Autodesk Inventor part; units mm, degrees
ref_plane "Work Plane1" through (0, 0, 10) normal (0, 0, 1) x (1, 0, 0)
ref_plane "YZ Plane" through (0, 0, 0) normal (1, 0, 0) x (0, 1, 0)
ref_plane "XZ Plane" through (0, 0, 0) normal (0, 1, 0) x (-1, 0, 0)
ref_plane "Work Plane1" through (0, 0, 10) normal (0, 0, 1) x (1, 0, 0)
sketch "Sketch1" plane through (0, 0, 10) normal (0, 0, 1) x (1, 0, 0)
  line L0 (-4.0299, -0.3538) -> (-2.2322, 1.4439) construction
  arc A0 (-1.4439, 2.2322) -> (-2.2322, 1.4439) centre (-0.9299, 0.9299) ccw construction
  line L1 (-1.4439, 2.2322) -> (0.3538, 4.0299) construction
  line L2 (-37.8299, 42.8299) -> (-37.8299, 37.8299) construction
  line L3 (-37.8299, 37.8299) -> (-42.9208, 37.8299) construction
  line L4 (-37.8299, 42.2137) -> (-37.8299, 45.8299) construction
  line L5 (-37.8299, 45.8299) -> (-4.0299, 45.8299) construction
  line L6 (-4.0299, 45.8299) -> (-4.0299, 42.2137) construction
  line L7 (-4.0299, 4.0299) -> (0.3538, 4.0299)
  circle A1 centre (-20.9299, 20.9299) radius 17.5
  line L8 (-20.9299, 58.9723) -> (17.1124, 20.9299) construction
  line L9 (17.1124, 20.9299) -> (-20.9299, -17.1124) construction
  line L10 (-20.9299, -17.1124) -> (-58.9723, 20.9299) construction
  line L11 (-58.9723, 20.9299) -> (-20.9299, 58.9723) construction
  line L12 (-20.9299, 58.9723) -> (-20.9299, -17.1124) construction
  line L13 (17.1124, 20.9299) -> (-58.9723, 20.9299) construction
  line L14 (-20.9299, 58.9723) -> (32.8701, 58.9723) construction
  line L15 (-43.4299, 43.4299) -> (1.5701, 43.4299) construction
  line L16 (1.5701, 43.4299) -> (1.5701, -1.5701) construction
  line L17 (1.5701, -1.5701) -> (-43.4299, -1.5701) construction
  line L18 (-43.4299, -1.5701) -> (-43.4299, 43.4299) construction
  line L19 (-43.4299, 43.4299) -> (1.5701, -1.5701) construction
  line L20 (1.5701, 43.4299) -> (-43.4299, -1.5701) construction
  line L21 (-43.4299, 5.3876) -> (-43.4299, 36.4723)
  line L22 (-43.4299, 36.4723) -> (-36.4723, 43.4299)
  line L23 (-36.4723, 43.4299) -> (-5.3876, 43.4299)
  line L24 (-5.3876, 43.4299) -> (1.5701, 36.4723)
  line L25 (1.5701, 36.4723) -> (1.5701, 5.3876)
  line L26 (1.5701, 5.3876) -> (-5.3876, -1.5701)
  line L27 (-5.3876, -1.5701) -> (-36.4723, -1.5701)
  line L28 (-36.4723, -1.5701) -> (-43.4299, 5.3876)
  line L29 (-4.0299, 42.2137) -> (-37.8299, 42.2137)
  line L30 (-4.0299, -0.3538) -> (-4.0299, 4.0299)
  circle A2 centre (-20.9299, 20.9299) radius 1.5
  line L31 (-10.9299, 10.9299) -> (-30.9299, 10.9299) construction
  line L32 (-30.9299, 10.9299) -> (-30.9299, 30.9299) construction
  line L33 (-30.9299, 30.9299) -> (-10.9299, 30.9299) construction
  line L34 (-10.9299, 30.9299) -> (-10.9299, 10.9299) construction
  line L35 (-10.9299, 10.9299) -> (-30.9299, 30.9299) construction
  line L36 (-30.9299, 10.9299) -> (-10.9299, 30.9299) construction
  circle A3 centre (-30.9299, 30.9299) radius 1.4
  circle A4 centre (-30.9299, 10.9299) radius 1.4
  circle A5 centre (-10.9299, 10.9299) radius 1.4
  line L37 (-45.8299, 37.8299) -> (-42.0723, 37.8299) construction
  line L38 (-42.1723, 37.7299) -> (-45.8299, 37.7299)
  line L39 (-45.8299, 37.7299) -> (-45.8299, 4.1299)
  line L40 (-45.8299, 4.1299) -> (-42.1723, 4.1299)
  line L41 (-42.1723, 4.1299) -> (-42.1723, 37.7299)
  line L42 (-45.8299, 4.0299) -> (-42.0723, 4.0299) construction
  line L43 (-45.8299, 37.8299) -> (-42.0723, 37.8299)
  line L44 (-37.7299, 45.8299) -> (-4.1299, 45.8299)
  line L45 (-4.1299, 45.8299) -> (-4.1299, 42.1723)
  line L46 (-4.1299, 42.1723) -> (-37.7299, 42.1723)
  line L47 (-37.7299, 42.1723) -> (-37.7299, 45.8299)
  line L48 (0.4701, 37.8299) -> (0.4701, 4.0299) construction
  line L49 (0.4701, 4.0299) -> (3.9701, 4.0299) construction
  line L50 (3.9701, 37.8299) -> (3.9701, 4.0299) construction
  line L51 (0.4701, 37.8299) -> (3.9701, 37.8299) construction
  line L52 (-45.8299, -3.9701) -> (-4.0299, -3.9701) construction
  line L53 (0.3124, 37.7299) -> (3.9701, 37.7299)
  line L54 (3.9701, 37.7299) -> (3.9701, 4.1299)
  line L55 (3.9701, 4.1299) -> (0.3124, 4.1299)
  line L56 (0.3124, 4.1299) -> (0.3124, 37.7299)
  line L57 (-4.1713, -0.3538) -> (-37.7299, -0.3538)
  line L58 (-37.7299, -0.3538) -> (-37.7299, -3.9701)
  line L59 (-37.7299, -3.9701) -> (-4.1713, -3.9701)
  line L60 (-4.1713, -3.9701) -> (-4.1713, -0.3538)
  point P0 (-37.8299, 4.0299)
  dimension "d18" = 53.8
  dimension "d19" = 45
  dimension "d20" = 53.8
  dimension "d21" = 45
  dimension "d22" = 45
  dimension "d30" = 20
  dimension "d31" = 20
  dimension "d32" = 2.8
  dimension "d33" = 2.8
  dimension "d34" = 2.8
  dimension "d35" = 3
  dimension "d36" = 0.1
  dimension "d37" = 0.1
  dimension "d38" = 0.1
  dimension "d39" = 0.1
extrude "Extrusion1" add sketch "Sketch1" along normal blind 5 contours L30 L26 L57 L28 L41 L22 L46 L24 L56 L7 | L7 L26 L30 | L56 L24 L25 L26 | L26 L25 L24 L53 L54 L55 | L60 L59 L58 L57 L28 L27 L26 | L26 L27 L28 L57 | L46 L22 L29 L24 | L24 L29 L45 | L40 L39 L38 L22 L21 L28 | L28 L21 L22 L41 | L29 L22 L23 L24 | L24 L23 L22 L29 L47 L44 L45 | L47 L29 L22 | A1
sketch "Skizze4" plane through (0, 0, 15) normal (0, 0, 1) x (1, 0, 0)
  circle A0 centre (-10.9299, 10.9299) radius 1.4 construction
  circle A1 centre (-30.9299, 10.9299) radius 1.4 construction
  circle A2 centre (-30.9299, 30.9299) radius 1.4 construction
  circle A3 centre (-20.9299, 20.9299) radius 1.5 construction
  line L0 (-37.7299, 42.1723) -> (-42.1723, 37.7299)
  line L1 (-42.1723, 37.7299) -> (-45.8299, 37.7299)
  line L2 (-45.8299, 37.7299) -> (-45.8299, 4.1299) construction
  line L3 (-45.8299, 4.1299) -> (-42.1723, 4.1299)
  line L4 (-42.1723, 4.1299) -> (-37.6885, -0.3538)
  line L5 (-37.6885, -0.3538) -> (-37.7299, -0.3538)
  line L6 (-37.7299, -0.3538) -> (-37.7299, -3.9701)
  line L7 (-37.7299, -3.9701) -> (-4.1713, -3.9701) construction
  line L8 (-4.1713, -3.9701) -> (-4.1713, -0.3538)
  line L9 (-4.1713, -0.3538) -> (0.3124, 4.1299)
  line L10 (0.3124, 4.1299) -> (3.9701, 4.1299)
  line L11 (3.9701, 4.1299) -> (3.9701, 37.7299) construction
  line L12 (3.9701, 37.7299) -> (0.3124, 37.7299)
  line L13 (0.3124, 37.7299) -> (-4.1299, 42.1723)
  line L14 (-4.1299, 42.1723) -> (-4.1299, 45.8299)
  line L15 (-4.1299, 45.8299) -> (-37.7299, 45.8299) construction
  line L16 (-37.7299, 45.8299) -> (-37.7299, 42.1723)
  line L17 (-37.9299, 46.0299) -> (-3.9299, 46.0299) construction
  line L18 (-3.9299, 46.0299) -> (-3.9299, 42.2551)
  line L19 (-3.9299, 42.2551) -> (0.3953, 37.9299)
  line L20 (0.3953, 37.9299) -> (4.1701, 37.9299)
  line L21 (4.1701, 37.9299) -> (4.1701, 3.9299) construction
  line L22 (4.1701, 3.9299) -> (0.3953, 3.9299)
  line L23 (0.3953, 3.9299) -> (-3.9713, -0.4367)
  line L24 (-3.9713, -0.4367) -> (-3.9713, -4.1701)
  line L25 (-3.9713, -4.1701) -> (-37.9299, -4.1701) construction
  line L26 (-37.9299, -4.1701) -> (-37.9299, -0.3953)
  line L27 (-37.9299, -0.3953) -> (-42.2551, 3.9299)
  line L28 (-42.2551, 3.9299) -> (-46.0299, 3.9299)
  line L29 (-46.0299, 3.9299) -> (-46.0299, 37.9299) construction
  line L30 (-46.0299, 37.9299) -> (-42.2551, 37.9299)
  line L31 (-42.2551, 37.9299) -> (-37.9299, 42.2551)
  line L32 (-37.9299, 42.2551) -> (-37.9299, 46.0299)
  line L33 (-45.8299, 37.7299) -> (-45.8299, 37.9299)
  line L34 (-4.1299, 45.8299) -> (-37.7299, 45.8299)
  line L35 (-37.7299, 45.8299) -> (-37.9299, 45.8299)
  line L36 (-4.1299, 45.8299) -> (-3.9299, 45.8299)
  line L37 (3.9701, 37.7299) -> (3.9701, 37.9299)
  line L38 (3.9701, 4.1299) -> (3.9701, 37.7299)
  line L39 (3.9701, 4.1299) -> (3.9701, 3.9299)
  line L40 (-4.1713, -3.9701) -> (-3.9713, -3.9701)
  line L41 (-37.7299, -3.9701) -> (-37.9299, -3.9701)
  line L42 (-45.8299, 4.1299) -> (-45.8299, 3.9299)
  point P0 (0, 0)
  dimension "d40" = 0.2
extrude "IM_offset" add sketch "Skizze4" against normal up to surface (5 mm away)
properties part number "20_Cube_Insert_Kinematic_Mirrormount_base_v3"
Can you work these out from the model? Positions are in its coordinate system, mm. A direction names the side the tool comes from. Coordinates: 2 decimals unless noted, no trailing zeros. Loops run counter-clockwise (first coordinate to the right, second up) from the corner with the lowest first, then second, coordinate; pieces in that order, holes last. Notation, with made-up numbers: (87, 18) - (105, 18) arc R24 cw to (105, 34) - close; hole circle Ø9 at (72, 80). An arc over 180 degrees is marked (long way). Put each result on its own line as item: value. Start each with the question number.
Item 1: Suppose I cut it at B-B (x = -31). Please give me the cut outline in (y, z), and give its area (3 significant figures).
Item 2: Which directions (+Z, -Z, +X, -X, +Y, -Y) give clear straight access to the entire face, cutting with the end or side of a thin tool? Please do faces 1 (the face through (-45.83, 21, 12)), 2 (the face through (-3.93, 44, 13)), 3 (the face through (-37.93, 44, 13)), 4 (the face through (-21, 27, 15)), 5 (the face through (-37.93, -2, 13)).
Item 3: If I drill on line 1 along Y through (x, z) = (-31, 13.3); line 2 along X through (y, z) = (43.5, 11.9); line 3 along Y through (x, z) = (-21.5, 13.4), over which ranges is the centre line in solid material (lowest first)?
Item 4: Suppose I cut it at C-C (z = 14.25). Please give me the cut outline in (x, y).
Item 5: For pin 1 (3 mm diameter, centred on x = 2.5, z = 11.5, fed in from +Y); pin 2 (3 mm diameter, centred on y = 43.5, z = 12, fed in from -X) (3 decimals); pin 3 (3 mm diameter, centred on y = 38.5, z = 13.5, fed in from +X); pin 4 (1.1 mm diameter, centred on y = -2.5, z = 13.5, fed in from -X), each with a flat end and sliding along its axis, tell me the tip position at first contact or that it passes through.
Item 6: Suppose I cut it at A-A (y = 21.5). Please give me the cut outline in (x, z).
Item 7: Suppose I cut it at D-D (x = -1.5). Please give me the cut outline in (y, z), and give its area (3 significant figures).
Item 8: If we mould it in two halves opening along Y, with no side actions, what happens to faces 6 (the face through (-44, 37.93, 13)), 7 (the face through (-29.595, 10.509, 12.465)), 8 (the face through (2, 3.93, 13))? For each: +Y half, -Y half, draft (parallel to the pull), parting line (faces both ways), or undercut.
Here are the results:
1. outline: (-3.97, 10) - (9.53, 10) - (9.53, 15) - (-3.97, 15) - close; (12.33, 10) - (29.53, 10) - (29.53, 15) - (12.33, 15) - close; (32.33, 10) - (45.83, 10) - (45.83, 15) - (32.33, 15) - close
1. area: 221 mm²
2. face 1: +Z, -Z, -X, +Y, -Y
2. face 2: +Z, -Z, +X, +Y
2. face 3: +Z, -Z, -X, +Y
2. face 4: +Z, +X, -X, +Y, -Y
2. face 5: +Z, -Z, -X, -Y
3. line 1: -3.97 to 9.53, 12.33 to 29.53, 32.33 to 45.83
3. line 2: -37.93 to -3.93
3. line 3: -3.97 to 19.54, 22.32 to 45.83
4. outline: (-45.83, 3.93) - (-42.26, 3.93) - (-37.93, -0.4) - (-37.93, -3.97) - (-3.97, -3.97) - (-3.97, -0.44) - (0.4, 3.93) - (3.97, 3.93) - (3.97, 37.93) - (0.4, 37.93) - (-3.93, 42.26) - (-3.93, 45.83) - (-37.93, 45.83) - (-37.93, 42.26) - (-42.26, 37.93) - (-45.83, 37.93) - close; hole circle Ø2.8 at (-30.93, 10.93); hole circle Ø2.8 at (-30.93, 30.93); hole circle Ø3 at (-20.93, 20.93); hole circle Ø2.8 at (-10.93, 10.93)
5. pin 1: y = 37.93
5. pin 2: x = -38.185
5. pin 3: x = 3.97
5. pin 4: x = -37.93
6. outline: (-45.83, 10) - (-22.32, 10) - (-22.32, 15) - (-45.83, 15) - close; (-19.54, 10) - (3.97, 10) - (3.97, 15) - (-19.54, 15) - close
7. outline: (2.03, 10) - (39.83, 10) - (39.83, 15) - (2.03, 15) - close
7. area: 189 mm²
8. face 6: +Y half
8. face 7: undercut
8. face 8: -Y half
